Autodesk Inventor part; units mm, degrees
ref_plane "YZ Plane" through (0, 0, 0) normal (1, 0, 0) x (0, 1, 0)
ref_plane "XZ Plane" through (0, 0, 0) normal (0, 1, 0) x (-1, 0, 0)
ref_plane "XY Plane" through (0, 0, 0) normal (0, 0, 1) x (1, 0, 0)
sketch "Эскиз1" plane through (0, 0, 0) normal (0, 1, 0) x (-1, 0, 0)
  line L0 (-67.75, -52) -> (67.75, -52)
  line L1 (71.75, -48) -> (71.75, 48)
  line L2 (67.75, 52) -> (-67.75, 52)
  line L3 (-71.75, 48) -> (-71.75, -48)
  line L4 (-71.75, -52) -> (71.75, 52) construction
  line L5 (71.75, -52) -> (-71.75, 52) construction
  arc A0 (71.75, 48) -> (67.75, 52) centre (67.75, 48) ccw
  arc A1 (67.75, -52) -> (71.75, -48) centre (67.75, -48) ccw
  arc A2 (-71.75, -48) -> (-67.75, -52) centre (-67.75, -48) ccw
  arc A3 (-67.75, 52) -> (-71.75, 48) centre (-67.75, 48) ccw
  line L6 (185.8649, 102) -> (-116.75, 102)
  line L7 (-116.75, 102) -> (-116.75, -127)
  line L8 (-116.75, -127) -> (185.8649, -127)
  line L9 (185.8649, -127) -> (185.8649, 102)
  point P0 (0, 0)
  point P1 (34.5574, -127)
  dimension "d0" = 143.5
  dimension "d1" = 104
  dimension "d2" = 4
  dimension "d3" = 45
  dimension "d4" = 50
  dimension "d5" = 75
extrude "Выдавливание1" add sketch "Эскиз1" against normal blind 10
sketch "Эскиз2" plane through (-185.8649, 0, 102) normal (0, 0, 1) x (1, 0, 0)
  line L0 (0, 0) -> (302.6149, 0)
  line L1 (302.6149, 0) -> (343.2905, -46.792)
  line L2 (343.2905, -46.792) -> (0, -46.792)
  line L3 (0, 0) -> (0, -10)
  line L4 (0, -46.792) -> (0, 0)
  line L5 (0, 0) -> (302.6149, 0)
  line L6 (0, 0) -> (0, -10)
  line L7 (302.6149, -10) -> (0, -10)
  line L8 (302.6149, 0) -> (302.6149, -10)
  point P0 (185.8649, 0)
  point P1 (302.6149, 0)
  point P2 (0, -10)
  dimension "d8" = 131
  dimension "d9" = 62
extrude "Выдавливание2" add sketch "Эскиз2" against normal up to surface (229 mm away) contours L1 L2 L4 L7 L8
sketch "Эскиз3" plane through (116.75, 0, 102) normal (0.7547, 0.6561, 0) x (0, 0, -1)
  line L0 (56, -8.5) -> (148, -8.5)
  line L1 (152, -12.5) -> (152, -49.5)
  line L2 (148, -53.5) -> (56, -53.5)
  line L3 (52, -49.5) -> (52, -12.5)
  line L4 (0, 0) -> (229, 0)
  line L5 (154, 121.0429) -> (154, 32.1469)
  arc A0 (56, -8.5) -> (52, -12.5) centre (56, -12.5) ccw
  arc A1 (152, -12.5) -> (148, -8.5) centre (148, -12.5) ccw
  arc A2 (148, -53.5) -> (152, -49.5) centre (148, -49.5) ccw
  arc A3 (52, -49.5) -> (56, -53.5) centre (56, -49.5) ccw
  line L6 (102, -8.5) -> (102, -53.5)
  line L7 (150, 29.5227) -> (54, 29.5227)
  point P0 (102, 76.5949)
  point P1 (102, 29.5227)
  dimension "d12" = 100
  dimension "d13" = 45
  dimension "d14" = 8.5
  dimension "d16" = 4
extrude "Выдавливание3" cut sketch "Эскиз3" against normal blind 2
properties part number "3d"
Work out the finished part from the listing and answer in its coordinate system (mm). A direction names the side the tool comes from. Coordinates: 2 decimals unless noted, no trailing zeros. Write each loop counter-clockwise with the first axis right and the second up, starting at its lowest first coordinate (ties: lowest second). Pieces come first, ordered by that corner, then holes.
1. Consider line 1 along Y through (x, z) = (-22.5, -25); line 2 along Z through (x, y) = (-44, -4.5); line 3 along X through (y, z) = (-6.5, -40.5). Determine where each line is inside the solid, lowest interval first.
Results list:
line 1: y = -46.79 to -10
line 2: z = -127 to -52, 52 to 102
line 3: x = -185.86 to -71.75, 71.75 to 122.23
2. Flat-ended cylindrical pins translate along their axes: pin 1 (3 mm diameter, centred on y = -4.5, z = 2.5, fed in from +X); pin 2 (5 mm diameter, centred on y = -20.5, z = 41, fed in from +X); pin 3 (3 mm diameter, centred on y = -5.5, z = 67, fed in from +X) (3 decimals). Find the tip coordinate at first contact, or state that the pin passes through.
Results list:
pin 1: stops at x = 121.97
pin 2: stops at x = 134.09
pin 3: stops at x = 122.835
3. For faces 1 (the flat face through (-17, -23, 102)), 2 (the flat face through (71.75, -5, 1)), determine the directions among +Z, -Z, +X, -X, +Y, -Y from which every point of the face is accessible in a straight line to the end or side of a thin tool.
Results list:
face 1: +Z, +X, -X, +Y, -Y
face 2: +Y
4. The part is cut by section A-A, the plane z = 12. Write down the section's boundary in (x, y).
Results list:
outline: (-185.86, -46.79) - (157.43, -46.79) - (151.85, -40.38) - (150.34, -41.69) - (120.82, -7.73) - (122.33, -6.42) - (116.75, 0) - (71.75, 0) - (71.75, -10) - (-71.75, -10) - (-71.75, 0) - (-185.86, 0) - close
5. For a pull along Z with two mould halves and no side action, classify faces 3 (the flat face through (-12, -23, -127)), 4 (the flat face through (-185.865, -23, -14)), 5 (the flat face through (-1, -5, 52)) as +Z half, -Z half, draft (parallel to the pull), parting line (faces both ways), or undercut.
Results list:
face 3: -Z half
face 4: draft
face 5: undercut
6. The part is cut by section B-B, the plane x = -15. Write down the section's boundary in (y, z).
Results list:
outline: (-46.79, -127) - (0, -127) - (0, -52) - (-10, -52) - (-10, 52) - (0, 52) - (0, 102) - (-46.79, 102) - close
7. The part is cut by section D-D, the plane z = -80. Write down the section's boundary in (x, y), and give its area (3 significant figures).
Results list:
outline: (-185.86, -46.79) - (157.43, -46.79) - (116.75, 0) - (-185.86, 0) - close
area: 15,100 mm2
8. The part is cut by section C-C, the plane y = -26. Write down the section's boundary in (x, z), and give its area (3 significant figures).
Results list:
outline: (-185.86, -127) - (139.35, -127) - (139.35, -50) - (136.7, -50) - (136.7, 50) - (139.35, 50) - (139.35, 102) - (-185.86, 102) - close
area: 74,200 mm2
